Input: part model. Units: mm. Frame: model coordinates. Round coordinates to 2 decimals unless told otherwise and drop trailing zeros. Write each loop counter-clockwise with the first axis right and the second up, starting at its lowest first coordinate (ties: lowest second). Pieces come first, ordered by that corner, then holes. Notation, with made-up numbers: M 68.5,18 L 110.5,18 A36 ccw 110.5,53 Z; hole C 43.5,-35 d10. An arc over 180 degrees is marked long. Answer as CSV lines item,"result". Start each with the question number.
Autodesk Inventor part; units mm, degrees
ref_plane "YZ Plane" through (0, 0, 0) normal (1, 0, 0) x (0, 1, 0)
ref_plane "XZ Plane" through (0, 0, 0) normal (0, 1, 0) x (-1, 0, 0)
ref_plane "XY Plane" through (0, 0, 0) normal (0, 0, 1) x (1, 0, 0)
sketch "Sketch1" plane through (0, 0, 0) normal (0, 0, 1) x (1, 0, 0)
  line L0 (0, 0) -> (-4.9, 0)
  line L1 (-4.9, 0) -> (4.9, 0)
  line L2 (0, 0) -> (0, 5)
  line L3 (0, 5) -> (-2.5, 5)
  line L4 (-2.5, 5) -> (-4.9, 0)
  line L5 (0, 5) -> (2.5, 5)
  line L6 (2.5, 5) -> (4.9, 0)
  line L7 (0, 0) -> (0, 4)
  line L8 (0, 4) -> (-2.5, 4)
  line L9 (-2.5, 4) -> (-4.9, 0)
  line L10 (0, 4) -> (2.5, 4)
  line L11 (2.5, 4) -> (4.9, 0)
  line L12 (0, 4) -> (0, 5)
  line L13 (0, 4.5) -> (-2.5, 4.5)
  line L14 (-2.5, 4.5) -> (-4.9, 0)
  line L15 (0, 4.5) -> (2.5, 4.5)
  line L16 (2.5, 4.5) -> (4.9, 0)
  line L17 (-4.9, 0) -> (-2.2333, 5)
  line L18 (4.9, 0) -> (2.2333, 5)
  dimension "d0" = 4.9
  dimension "d1" = 9.8
  dimension "d5" = 5
  dimension "d6" = 2.5
  dimension "d7" = 2.5
  dimension "d33" = 4
extrude "Extrusion1" add sketch "Sketch1" along normal blind 50 contours L2 L10 L11 L1 | L0 L9 L8 L2 | L14 L13 L2 L8 L9 | L11 L10 L2 L15 L16 | L17 L3 L2 L13 | L15 L2 L5 L18
sketch "Sketch2" plane through (0, 0, 50) normal (0, 0, 1) x (1, 0, 0)
  line L0 (0, 5) -> (0, -65)
  circle A0 centre (0, -30) radius 35
  line L1 (-4.9, 0) -> (4.9, 0)
  line L2 (4.9, 0) -> (18.0278, 0)
  arc A1 (18.0278, 0) -> (2.5, 5) centre (2.5, -21.6111) ccw
  line L3 (4.9, 0) -> (0, 0)
  line L4 (2.5, 5) -> (0, 5)
  line L5 (-4.9, 0) -> (-18.0278, 0)
  arc A2 (-2.5, 5) -> (-18.0278, 0) centre (-2.5, -21.6111) ccw
  circle A3 centre (0, -30) radius 37.5
  line L6 (2.5, 6.0566) -> (32.476, -11.25)
  line L7 (32.476, -11.25) -> (32.476, -48.75)
  line L8 (32.476, -48.75) -> (0, -67.5)
  line L9 (0, -67.5) -> (-32.476, -48.75)
  line L10 (-32.476, -48.75) -> (-32.476, -11.25)
  line L11 (-32.476, -11.25) -> (-2.5, 6.0566)
  arc A4 (2.5, 6.0566) -> (-2.5, 6.0566) centre (0, 1.7265) ccw
  line L12 (-4.9, 0) -> (-12.9904, 0)
  line L13 (4.9, 0) -> (12.9904, 0)
  line L14 (4.9, 0) -> (-4.9, 0)
  circle A5 centre (0, -30) radius 30
  line L15 (-17.488, -2.5967) -> (0, -30)
  line L16 (0, -30) -> (17.488, -2.5967)
  circle A6 centre (0, -30) radius 32.508
  line L17 (0, -30) -> (-32.476, -11.25)
  line L18 (0, -30) -> (32.476, -11.25)
  arc A7 (-29.976, -9.8066) -> (-32.476, -14.1368) centre (-27.476, -14.1368) ccw
  arc A8 (-32.476, -45.8632) -> (-29.976, -50.1934) centre (-27.476, -45.8632) ccw
  arc A9 (-2.5, -66.0566) -> (2.5, -66.0566) centre (0, -61.7265) ccw
  arc A10 (29.976, -50.1934) -> (32.476, -45.8632) centre (27.476, -45.8632) ccw
  arc A11 (32.476, -14.1368) -> (29.976, -9.8066) centre (27.476, -14.1368) ccw
  line L19 (0, -30) -> (29.976, -9.8066)
  line L20 (2.5, 4.5) -> (-2.5, 4.5)
  line L21 (-2.5, 4.5) -> (-4.9, 0)
  line L22 (-2.5, 4.5) -> (-4.9, 0)
  line L23 (-4.9, 0) -> (-1.4228, 6.5198)
  point P0 (0, 0)
  point P1 (0, 0)
  point P2 (0, 7.5)
  point P3 (16.1388, -4.7109)
  point P4 (-16.1388, -4.7109)
  point P5 (-1.8396, 6.3758)
  point P6 (25.9808, -15)
  point P7 (-32.4222, -13.4053)
  point P8 (-30.5825, -49.7811)
  point P9 (1.8396, -66.3758)
  point P10 (32.4222, -46.5947)
  point P11 (30.5825, -10.2189)
  point P12 (24.881, -13.2389)
  point P13 (29.976, -9.8066)
  point P14 (-0.9147, 6.6421)
  point P15 (0, 4.5)
  dimension "d13" = 75
  dimension "d14" = 5
  dimension "d28" = 360
extrude "Extrusion2" [suppressed]
fillet "Fillet1" [suppressed]
chamfer "Chamfer4" distance 1 angle 45 2 edges at (4.9, 0, 25) (-4.9, 0, 25)
sketch "Sketch4" plane through (0, 0, 50) normal (0, 0, 1) x (1, 0, 0)
  line L0 (-14.1632, 12.0021) -> (30.9274, 12.0021)
  line L1 (30.9274, 12.0021) -> (30.9274, -18.7889)
  line L2 (30.9274, -18.7889) -> (-14.1632, -18.7889)
  line L3 (-14.1632, -18.7889) -> (-14.1632, 12.0021)
  line L4 (-3.9, 0) -> (-4.4294, 0.8824)
  line L5 (-3.9, 0) -> (-4.4294, 0.8824)
  line L6 (-2.5, 4.5) -> (-4.4294, 0.8824)
  line L7 (-4.4294, 0.8824) -> (-2.5, 4.5)
  line L8 (2.5, 4.5) -> (-2.5, 4.5)
  line L9 (-2.5, 4.5) -> (2.5, 4.5)
  line L10 (-3.9, 0) -> (0, 0)
  line L11 (3.9, 0) -> (-3.9, 0)
  line L12 (3.9, 0) -> (4.4294, 0.8824)
  line L13 (3.9, 0) -> (4.4294, 0.8824)
  line L14 (4.4294, 0.8824) -> (2.5, 4.5)
  line L15 (4.4294, 0.8824) -> (2.5, 4.5)
  line L16 (2.2333, 5) -> (4.4294, 0.8824)
  line L17 (-2.2333, 5) -> (2.2333, 5)
  line L18 (-1.4228, 6.5198) -> (-4.4294, 0.8824)
extrude "Extrusion3" cut sketch "Sketch4" against normal blind 7.5
properties part number "dishHolderArm_3DPrint"
Item 1: Cut plane B-B, the plane z = 26. Return loops of the section in (x, y).
Item 2: Line query: line 1 (X direction, y = 0.65, z = 10.5); line 2 (Y direction, x = 3.75, z = 32); line 3 (X direction, y = 0.8, z = 13). Output: solid intervals per line, ascending. Write a range as [from, to].
Item 3: Cut plane C-C, the plane y = 4. Return loops of the section in (x, z).
Item 4: Cut plane A-A, the plane y = 1.8. Return loops of the section in (x, z), plus the area to 3 significant figures.
Results list:
1,outline,"M -4.43,0.88 L -3.9,0 L 3.9,0 L 4.43,0.88 L 2.5,4.5 L 2.23,5 L -2.23,5 L -2.5,4.5 Z"
2,line 1,"[-4.29, 4.29]"
2,line 2,"[0, 2.16]"
2,line 3,"[-4.38, 4.38]"
3,outline,"M -2.77,0 L 2.77,0 L 2.77,50 L -2.77,50 Z"
4,outline,"M -3.94,0 L 3.94,0 L 3.94,50 L -3.94,50 Z"
4,area,"394 mm²"
